The listing builds one solid part. Answer for the finished solid, in the listing's coordinates (mm). Face numbers are marked on the shaded views. Give positions to 0.01 mm unless a question says otherwise; leave off trailing zeros. Order: outer loops, then holes, each group sorted by start corner. A loop starts at its lowest first (then second) coordinate and runs counter-clockwise, first axis right, second up. Notation, with made-up numbers: (0, 27) -> (17, 27) arc R6 ccw to (17, 34) -> close; hole circle Ø9 at (-0.5, -8). An arc over 180 degrees is marked (long way). Answer as a JSON object with one key per item and string values. Group by question number.
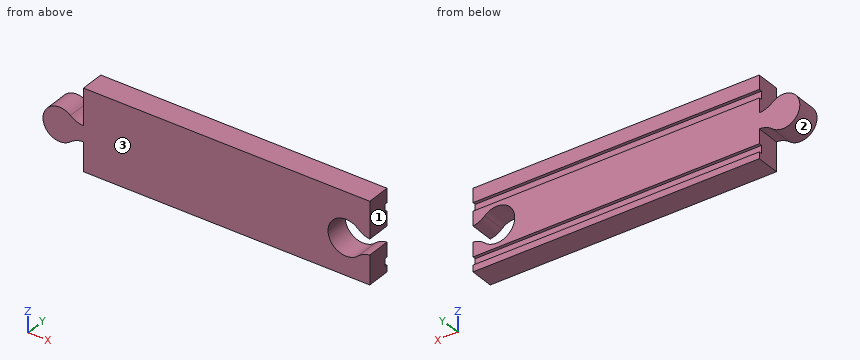
Autodesk Inventor part; units mm, degrees
ref_plane "YZ Plane" through (0, 0, 0) normal (1, 0, 0) x (0, 1, 0)
ref_plane "XZ Plane" through (0, 0, 0) normal (0, 1, 0) x (-1, 0, 0)
ref_plane "XY Plane" through (0, 0, 0) normal (0, 0, 1) x (1, 0, 0)
sketch "Sketch1" plane through (0, 0, 0) normal (0, 1, 0) x (-1, 0, 0)
  line L0 (0, 0) -> (304.8, 0)
  line L1 (304.8, 0) -> (304.8, -86.36)
  line L2 (304.8, -86.36) -> (0, -86.36)
  line L3 (0, -86.36) -> (0, 0)
  circle A0 centre (25.4, -47.2363) radius 19.05
  circle A1 centre (330.2, -47.2363) radius 17.78
  line L4 (34.5288, -55.4913) -> (0, -55.4913)
  line L5 (34.5288, -38.9813) -> (0, -38.9813)
  line L6 (34.5288, -38.9813) -> (34.5288, -55.4913)
  line L7 (0, -38.9813) -> (0, -55.4913)
  line L8 (331.681, -55.4913) -> (282.1836, -55.4913)
  line L9 (331.681, -38.9813) -> (282.1836, -38.9813)
  line L10 (331.681, -38.9813) -> (331.681, -55.4913)
  line L11 (282.1836, -38.9813) -> (282.1836, -55.4913)
  dimension "d0" = 304.8
  dimension "d1" = 86.36
extrude "Extrusion1" add sketch "Sketch1" along normal blind 25.4
extrude "Extrusion2" cut sketch "Sketch1" along normal blind 25.4 contours L5 A0 L4 L3 | L5 L6 L4 A0 | A0 L4 L6 L5
fillet "Fillet1" radius 22.86 4 edges at (-8.2315, 12.7, -55.4913) (-8.2315, 12.7, -38.9813) (-314.4525, 12.7, -38.9813) (-314.4525, 12.7, -55.4913)
sketch "Sketch2" plane through (0, 0, 0) normal (1, 0, 0) x (0, 0, -1)
  line L0 (38.9813, 25.4) -> (0, 25.4)
  line L1 (14.8709, 25.4) -> (23.7033, 25.4)
  line L2 (23.7033, 25.4) -> (23.7033, 22.0925)
  line L3 (23.7033, 22.0925) -> (14.8709, 22.0925)
  line L4 (14.8709, 22.0925) -> (14.8709, 25.4)
  line L5 (86.36, 25.4) -> (55.4913, 25.4)
  line L6 (70.9256, 25.4) -> (79.3317, 25.4)
  line L7 (79.3317, 25.4) -> (79.3317, 22.0925)
  line L8 (79.3317, 22.0925) -> (70.9256, 22.0925)
  line L9 (70.9256, 22.0925) -> (70.9256, 25.4)
  point P0 (0, 0)
extrude "Extrusion3" cut sketch "Sketch2" against normal blind 379.4125
properties part number "train track"
(1) A cutting plane is placed at D-D (x = -330.2). Determine the outline of the cut face in (y, z), and give its area (3 significant figures).
(2) A cutting plane is placed at C-C (y = 12.75). Determine the outline of the cut face in (x, z).
(3) A cutting plane is placed at B-B (x = -81.5). Determine the outline of the cut face in (y, z).
(4) For a pull along X with two mould halves and no side action, classify the marked faces 1, 2 and 3 as +X half, -X half, draft (parallel to the pull), parting line (faces both ways), or undercut.
(5) Flat-ended cylindrical pins translate along their axes: pin 1 Ø7.5 at (y, z) = (12.5, -73) entering from -X; pin 2 Ø6.5 at (x, z) = (-185.5, -76) entering from +Y. Find the tip coordinate at first contact, or state that the pin passes through.
(6) A cutting plane is placed at A-A (x = -25.4). Determine the outline of the cut face in (y, z), and give its area (3 significant figures).
(7) Find the intervals of material crossed by line 1 along Z through (x, y) = (-25.4, 8.25); line 2 along X through (y, z) = (23.25, -46); line 3 along X through (y, z) = (21.5, -74), in increasing order. Write a range as [from, to].
Check sheet entries:
{
 "1": {"outline": "(0, -65.02) -> (25.4, -65.02) -> (25.4, -29.46) -> (0, -29.46) -> close", "area": "903 mm2"},
 "2": {"outline": "(-318.76, -60.84) arc R22.86 cw to (-304.8, -55.49) -> (-304.8, -86.36) -> (0, -86.36) -> (0, -55.49) arc R22.86 ccw to (-12.55, -61.3) arc R19.05 cw (long way) to (-12.55, -33.18) arc R22.86 ccw to (0, -38.98) -> (0, 0) -> (-304.8, 0) -> (-304.8, -38.98) arc R22.86 cw to (-318.76, -33.63) arc R17.78 ccw (long way) to start"},
 "3": {"outline": "(0, -86.36) -> (25.4, -86.36) -> (25.4, -79.33) -> (22.09, -79.33) -> (22.09, -70.93) -> (25.4, -70.93) -> (25.4, -23.7) -> (22.09, -23.7) -> (22.09, -14.87) -> (25.4, -14.87) -> (25.4, 0) -> (0, 0) -> close"},
 "4": {"face 1": "+X half", "face 2": "undercut", "face 3": "draft"},
 "5": {"pin 1": "stops at x = -304.8", "pin 2": "stops at y = 22.09"},
 "6": {"outline": "(0, -86.36) -> (25.4, -86.36) -> (25.4, -79.33) -> (22.09, -79.33) -> (22.09, -70.93) -> (25.4, -70.93) -> (25.4, -66.29) -> (0, -66.29) -> close; (0, -28.19) -> (25.4, -28.19) -> (25.4, -23.7) -> (22.09, -23.7) -> (22.09, -14.87) -> (25.4, -14.87) -> (25.4, 0) -> (0, 0) -> close", "area": "1,170 mm2"},
 "7": {"line 1": "z = [-86.36, -66.29], [-28.19, 0]", "line 2": "x = [-347.94, -44.41]", "line 3": "x = [-304.8, 0]"}
}
